Design review of the part built by this model. Coordinates are the model's own, in mm. A direction names the side the tool comes from. Give positions to 0.01 mm unless a question says otherwise; leave off trailing zeros. Loops run counter-clockwise (first coordinate to the right, second up) from the corner with the lowest first, then second, coordinate; pieces in that order, holes last.
from build123d import *

# Parameters (mm, degrees)
SKETCH2_R                            = 3.2385
BOSS_EXTRUDE1_DEPTH                  = 6.0198
BOSS_EXTRUDE5_DEPTH                  = 4.4958
SKETCH5_R                            = 1.9812
CUT_EXTRUDE2_ENCODERSCREWHOLES_DEPTH = 40.704494042
CUT_EXTRUDE4_DEPTH                   = 2.8448
SKETCH13_R                           = 1.5875
CUT_EXTRUDE5_DEPTH                   = 40.704494042
SKETCH7_R                            = 3.96875
BOSS_EXTRUDE4_DEPTH                  = 3.175
SKETCH14_R                           = 3.175
CUT_EXTRUDE6_DEPTH                   = 41.629874457


with BuildPart() as part:
    # Sketch2 → Boss-Extrude1 (new body)
    with BuildSketch(Plane.XY):
        with BuildLine():
            Line((14.3891, -36.5125), (-14.3891, -36.5125))
            Line((-14.3891, -36.5125), (-14.3891, 11.742361964))
            ThreePointArc((-14.3891, 11.742361964), (0, 18.5166), (14.3891, 11.742361964))
            Line((14.3891, 11.742361964), (14.3891, -36.5125))
        make_face()
        Circle(SKETCH2_R, mode=Mode.SUBTRACT)
    extrude(amount=BOSS_EXTRUDE1_DEPTH)

    # Sketch12 → Boss-Extrude5 (add)
    with BuildSketch(Plane.XY.offset(6.0198)):
        with BuildLine():
            Line((-14.3891, 6.247076947), (-14.3891, 11.742361964))
            ThreePointArc((-14.3891, 11.742361964), (0, 18.5166), (14.3891, 11.742361964))
            Line((14.3891, 11.742361964), (14.3891, 6.247076947))
            ThreePointArc((14.3891, 6.247076947), (0, 15.5956), (-14.3891, 6.247076947))
        make_face()
    extrude(amount=BOSS_EXTRUDE5_DEPTH)

    # Sketch5 → Cut-Extrude2_EncoderScrewHoles (cut, through all)
    with BuildSketch(Plane.XY.offset(6.0198)):
        with Locations((-9.525, 0)):
            Circle(SKETCH5_R)
        with Locations((9.525, 0)):
            Circle(SKETCH5_R)
    extrude(amount=-CUT_EXTRUDE2_ENCODERSCREWHOLES_DEPTH, mode=Mode.SUBTRACT)

    # Sketch11 → Cut-Extrude4 (cut)
    with BuildSketch(Plane(origin=(0, 0, 0), x_dir=(-1, 0, 0), z_dir=(0, 0, -1))):
        Polygon((9.525, -3.372880273), (12.446, -1.686440136), (12.446, 1.686440136), (9.525, 3.372880273), (6.604, 1.686440136), (6.604, -1.686440136), align=None)
        Polygon((-6.604, -1.686440136), (-6.604, 1.686440136), (-9.525, 3.372880273), (-12.446, 1.686440136), (-12.446, -1.686440136), (-9.525, -3.372880273), align=None)
    extrude(amount=-CUT_EXTRUDE4_DEPTH, mode=Mode.SUBTRACT)

    # Sketch13 → Cut-Extrude5 (cut, through all)
    with BuildSketch(Plane.XY.offset(6.0198)):
        with Locations((8.89, -31.75)):
            Circle(SKETCH13_R)
        with Locations((-8.89, -31.75)):
            Circle(SKETCH13_R)
    extrude(amount=-CUT_EXTRUDE5_DEPTH, mode=Mode.SUBTRACT)

    # Sketch7 → Boss-Extrude4 (add)
    with BuildSketch(Plane(origin=(0, 0, 0), x_dir=(-1, 0, 0), z_dir=(0, 0, -1))):
        with Locations((0, -15.875)):
            Circle(SKETCH7_R)
    extrude(amount=BOSS_EXTRUDE4_DEPTH)

    # Sketch14 → Cut-Extrude6 (cut, through all)
    with BuildSketch(Plane(origin=(0, 0, 0), x_dir=(-1, 0, 0), z_dir=(0, 0, -1))):
        with Locations((0, 11.1125)):
            Circle(SKETCH14_R)
    extrude(amount=-CUT_EXTRUDE6_DEPTH, mode=Mode.SUBTRACT)


solid = part.part
Q1. Tool access review of faces 1 (the face through (-6.604, 0, 1)), 2 (the face through (1, 16, 10.516)), 3 (the face through (0, -10, 6.02)): name each direction out of +Z, -Z, +X, -X, +Y, -Y from which nothing blocks a thin tool from reaching the whole face with its end or side.
Results:
face 1: -Z
face 2: +Z, +X, -X, +Y, -Y
face 3: +Z, -Y
Q2. Draft analysis for pull direction Y (two halves, no side actions). For faces 4 (the face through (0, -9, 0)), 5 (the face through (6.604, 0, 1)), 6 (the face through (-0.23, 18.515, 5.184)), state which applies: pulls with the +Y half, pulls with the -Y half, needs draft (parallel to the pull), parting line crosses it, or undercut.
Results:
face 4: needs draft
face 5: undercut
face 6: pulls with the +Y half
Q3. Insertion check: pin 1 (10 mm diameter, centred on x = 0, y = 11.11, fed in from -Z); pin 2 (2 mm diameter, centred on x = -1.5, y = 0.5, fed in from +Z); pin 3 (6 mm diameter, centred on x = 11, y = -0.5, fed in from +Z); pin 4 (4 mm diameter, centred on y = 4, z = -1.5, fed in from +X). Each pin has a flat end and moves straight along its axis. Give the tip position at first contact, or say it passes through.
Results:
pin 1: stops at z = 0
pin 2: passes through
pin 3: stops at z = 6.02
pin 4: stops at x = 14.39
Q4. Take a section at D-D (y = 12.5). Give the boundary of the cut face in (x, z), plus the area to 3 significant figures.
Results:
outline: (-13.73, 0) - (-2.86, 0) - (-2.86, 6.02) - (-9.38, 6.02) - (-9.38, 10.52) - (-13.73, 10.52) - close; (2.86, 0) - (13.73, 0) - (13.73, 10.52) - (9.38, 10.52) - (9.38, 6.02) - (2.86, 6.02) - close
area: 170 mm2
Q5. Take a section at B-B (x = 0). Give the boundary of the cut face in (y, z) (1 decimal), plus the area to 3 significant figures.
Results:
outline: (-36.5, 0) - (-19.8, 0) - (-19.8, -3.2) - (-11.9, -3.2) - (-11.9, 0) - (-3.2, 0) - (-3.2, 6) - (-36.5, 6) - close; (3.2, 0) - (7.9, 0) - (7.9, 6) - (3.2, 6) - close; (14.3, 0) - (18.5, 0) - (18.5, 10.5) - (15.6, 10.5) - (15.6, 6) - (14.3, 6) - close
area: 292 mm2
Q6. Wall thickness on line 1 (Y direction, x = 0, z = 4.75); line 2 (Z direction, x = 11.5, y = -30.5); line 3 (Y direction, x = 8.89, z = 2.75): over which ranges is each line inside the solid? List them lowest first.
Results:
line 1: y = -36.51 to -3.24, 3.24 to 7.94, 14.29 to 18.52
line 2: z = 0 to 6.02
line 3: y = -36.51 to -33.34, -30.16 to -3.01, 3.01 to 16.26
Q7. Take a section at C-C (y = -31.75). Give the boundary of the cut face in (x, z), plus the area to 3 significant figures.
Results:
outline: (-14.39, 0) - (-10.48, 0) - (-10.48, 6.02) - (-14.39, 6.02) - close; (-7.3, 0) - (7.3, 0) - (7.3, 6.02) - (-7.3, 6.02) - close; (10.48, 0) - (14.39, 0) - (14.39, 6.02) - (10.48, 6.02) - close
area: 135 mm2
Q8. Take a section at A-A (y = 0). Give the boundary of the cut face in (x, z).
Results:
outline: (-14.39, 0) - (-12.45, 0) - (-12.45, 2.84) - (-11.51, 2.84) - (-11.51, 6.02) - (-14.39, 6.02) - close; (-7.54, 2.84) - (-6.6, 2.84) - (-6.6, 0) - (-3.24, 0) - (-3.24, 6.02) - (-7.54, 6.02) - close; (3.24, 0) - (6.6, 0) - (6.6, 2.84) - (7.54, 2.84) - (7.54, 6.02) - (3.24, 6.02) - close; (11.51, 2.84) - (12.45, 2.84) - (12.45, 0) - (14.39, 0) - (14.39, 6.02) - (11.51, 6.02) - close
